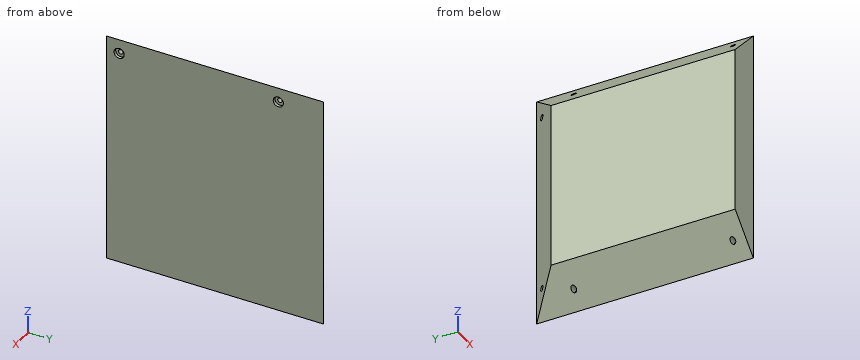
```python
from build123d import *

# Parameters (mm, degrees)
SKETCH1_W                               = 300
SKETCH1_H                               = 260
BOSS_EXTRUDE1_DEPTH                     = 39
CUT_EXTRUDE1_DEPTH                      = 260
CUT_EXTRUDE2_DEPTH                      = 384
F_6_0MM_DOWEL_HOLE1_D                   = 6
F_6_0MM_DOWEL_HOLE1_DEPTH               = 30
F_6_0MM_DOWEL_HOLE1_TIP                 = 1.802581857
CBORE_FOR_M5_HEX_HEAD_BOLT1_D           = 5.5
CBORE_FOR_M5_HEX_HEAD_BOLT1_DEPTH       = 30
CBORE_FOR_M5_HEX_HEAD_BOLT1_CBORE_D     = 12.238
CBORE_FOR_M5_HEX_HEAD_BOLT1_CBORE_DEPTH = 3.5
CBORE_FOR_M5_HEX_HEAD_BOLT1_TIP         = 1.652366702
F_6_0MM_DOWEL_HOLE2_D                   = 6
F_6_0MM_DOWEL_HOLE2_DEPTH               = 30
F_6_0MM_DOWEL_HOLE2_TIP                 = 1.802581857


with BuildPart() as part:
    # Sketch1 → Boss-Extrude1 (new body)
    with BuildSketch(Plane(origin=(0, 0, 0), x_dir=(0, 0, -1), z_dir=(1, 0, 0))):
        Rectangle(SKETCH1_W, SKETCH1_H)
    extrude(amount=BOSS_EXTRUDE1_DEPTH)

    # Sketch3 → Cut-Extrude1 (cut)
    with BuildSketch(Plane(origin=(0, -130, 0), x_dir=(-1, 0, 0), z_dir=(0, -1, 0))):
        Polygon((-39, 150), (0, 150), (0, 111), align=None)
        Polygon((0, -127.51), (0, -88.51), (-39, -127.51), (-39, -150), (0, -150), align=None)
    extrude(amount=-CUT_EXTRUDE1_DEPTH, mode=Mode.SUBTRACT)

    # Sketch5 → Cut-Extrude2 (cut)
    with BuildSketch(Plane(origin=(0, 0, -150), x_dir=(-1, 0, 0), z_dir=(0, 0, -1))):
        Polygon((-39, 130), (0, 130), (0, 91), align=None)
    extrude(amount=-CUT_EXTRUDE2_DEPTH, mode=Mode.SUBTRACT)

    # Ø6.0mm Dowel Hole1
    with Locations(Plane.ZY):
        with Locations((-133, -115), (-133, 76)):
            Hole(F_6_0MM_DOWEL_HOLE1_D / 2, depth=F_6_0MM_DOWEL_HOLE1_DEPTH)
            with Locations((0, 0, -(F_6_0MM_DOWEL_HOLE1_DEPTH + F_6_0MM_DOWEL_HOLE1_TIP / 2))):  # 118° drill point
                Cone(0, F_6_0MM_DOWEL_HOLE1_D / 2, F_6_0MM_DOWEL_HOLE1_TIP, mode=Mode.SUBTRACT)

    # CBORE for M5 Hex Head Bolt1
    with Locations(Plane(origin=(39, 0, 0), x_dir=(0, 0, -1), z_dir=(1, 0, 0))):
        with Locations((-110.51, -115), (-110.51, 76)):
            CounterBoreHole(CBORE_FOR_M5_HEX_HEAD_BOLT1_D / 2, CBORE_FOR_M5_HEX_HEAD_BOLT1_CBORE_D / 2, CBORE_FOR_M5_HEX_HEAD_BOLT1_CBORE_DEPTH, depth=CBORE_FOR_M5_HEX_HEAD_BOLT1_DEPTH)
            with Locations((0, 0, -(CBORE_FOR_M5_HEX_HEAD_BOLT1_DEPTH + CBORE_FOR_M5_HEX_HEAD_BOLT1_TIP / 2))):  # 118° drill point
                Cone(0, CBORE_FOR_M5_HEX_HEAD_BOLT1_D / 2, CBORE_FOR_M5_HEX_HEAD_BOLT1_TIP, mode=Mode.SUBTRACT)

    # Ø6.0mm Dowel Hole2
    with Locations(Plane(origin=(0, 130, 0), x_dir=(1, 0, 0), z_dir=(0, 1, 0))):
        with Locations((25, -95.51), (25, 118)):
            Hole(F_6_0MM_DOWEL_HOLE2_D / 2, depth=F_6_0MM_DOWEL_HOLE2_DEPTH)
            with Locations((0, 0, -(F_6_0MM_DOWEL_HOLE2_DEPTH + F_6_0MM_DOWEL_HOLE2_TIP / 2))):  # 118° drill point
                Cone(0, F_6_0MM_DOWEL_HOLE2_D / 2, F_6_0MM_DOWEL_HOLE2_TIP, mode=Mode.SUBTRACT)


solid = part.part
```
Input: part model. Units: mm. Frame: model coordinates. Coordinates: 2 decimals unless noted, no trailing zeros. Loops run counter-clockwise (first coordinate to the right, second up) from the corner with the lowest first, then second, coordinate; pieces in that order, holes last. Notation, with made-up numbers: M -19,41.25 L 17,41.25 A23 cw 17,80.25 Z; hole C 12,3 d10. An arc over 180 degrees is marked long. Use a Markdown table: item, result. Add a question column.
1) Section B-B, the plane y = 49. Return the cut outline in (x, z).
2) Section A-A, the plane x = 11.5. Return the cut outline in (y, z).
3) Line query: L1, parallel to Z at x = 29.25, y = -115; L2, parallel to Y at x = 37.5, z = 115.5; L3, parallel to Y at x = 37, z = 110. Output: solid intervals per line, ascending. Write a range as from..to.
4) Pin query (flat end, axial travel): P1, Ø3, axis at x = 26, y = -11.5, coming from the +Z side; P2, Ø4, axis at x = 6, y = -84, coming from the -Z side; P3, Ø6, axis at y = 73.5, z = 109, coming from the +X side; P4, Ø10, axis at y = -115, z = 109, coming from the +X side. Return the tip coordinate at first contact, or that it passes through.
Answer below:
| question | item | result |
|---|---|---|
| 1 | outline | M 0,-111 L 39,-150 L 39,127.51 L 0,88.51 Z |
| 2 | outline | M -130,-122.5 L 102.5,-122.5 L 102.5,100.01 L -130,100.01 Z |
| 3 | L1 | -140.25..-136, -130..107.76, 113.26..117.76 |
| 3 | L2 | -130..-118.54, -111.46..72.46, 79.54..128.5 |
| 3 | L3 | -130..-121.1, -108.9..69.9, 82.1..128 |
| 4 | P1 | z = 116.01 |
| 4 | P2 | z = -119 |
| 4 | P3 | x = 35.5 |
| 4 | P4 | x = 39 |
